```python
from build123d import *

# Parameters (mm, degrees)
F0_W          = 39
F0_H          = 51
F1_DEPTH      = 6
F2_R          = 1.4383077573
F3_DEPTH      = 4
F3_DEPTH_BACK = 4
F5_DEPTH      = 2
F6_W          = 39
F6_H          = 2.9835407734
F6_H_2        = 3.1214025915
F7_DEPTH      = 37
F8_SIZE       = 7
F9_T1_DEPTH   = 61
F10_W         = 13
F10_H         = 22
F11_DEPTH     = 15.8


# Not quite as in the source:
# - a fillet or chamfer that OpenCascade refuses, or shapes differently, is made with other operations: its cross-section is extruded or revolved along the edge and cut away or added
# - a pattern or mirror of a feature is missing from the dataset's text; its kind, count and spacing are read off the source's solid


with BuildPart() as f1:
    # F0 (on Top) → F1 (new body)
    with BuildSketch(Plane.XY):
        Rectangle(F0_W, F0_H)
    extrude(amount=F1_DEPTH)

    # F2 (on Front) → F3 (join, two sides)
    with BuildSketch(Plane.XZ) as f3_sk:
        with BuildLine():
            Line((-2.7218379916, 29.2536051472), (-13.5, 6))
            Line((-13.5, 6), (13.5, 6))
            Line((13.5, 6), (2.7218379916, 29.2536051472))
            ThreePointArc((2.7218379916, 29.2536051472), (0, 30.9920196576), (-2.7218379916, 29.2536051472))
        make_face()
        with Locations((0, 27.9920196576)):
            Circle(F2_R, mode=Mode.SUBTRACT)
    extrude(amount=F3_DEPTH)
    extrude(f3_sk.sketch, amount=-F3_DEPTH_BACK)

    # F4 (on face) → F5 (cut)
    with BuildSketch(Plane.XZ.offset(4)):
        with BuildLine():
            Line((-2.3500163027, 26.2716104284), (-11.7460088804, 6))
            Line((-11.7460088804, 6), (11.7170447484, 6))
            Line((11.7170447484, 6), (2.3322070272, 26.2475441144))
            ThreePointArc((2.3322070272, 26.2475441144), (-0.0149696172, 25.0796047749), (-2.3500163027, 26.2716104284))
        make_face()
    f5 = extrude(amount=-F5_DEPTH, mode=Mode.SUBTRACT)

    # F5_copies: F5 across plane
    add(f5.mirror(Plane.ZX), mode=Mode.SUBTRACT)

    # F6 (on face) → F7 (join)
    with BuildSketch(Plane.XY.offset(6)):
        with Locations((0, 24.0082296133)):
            Rectangle(F6_W, F6_H)
        with Locations((0, -23.9392987043)):
            Rectangle(F6_W, F6_H_2)
    extrude(amount=F7_DEPTH)

    # F8
    f8_edges = [f1.edges().sort_by_distance(p)[0] for p in [
        (19.5, 24.00823, 43),
        (-19.5, 24.00823, 43),
        (-19.5, -23.939299, 43),
        (19.5, -23.939299, 43),
    ]]
    chamfer(f8_edges, length=F8_SIZE)

    # F9: fillet of radius 5 on 4 edges, made by hand

    # F9_s2 → F9_t1 (cut)
    with BuildSketch(Plane.XY.offset(-12.5)):
        with BuildLine():
            ThreePointArc((19.5, -20.5), (18.0355339059, -24.0355339059), (14.5, -25.5))
            Line((14.5, -25.5), (19.5, -25.5))
            Line((19.5, -25.5), (19.5, -20.5))
        make_face()
        with BuildLine():
            ThreePointArc((-19.5, -20.5), (-18.0355339059, -24.0355339059), (-14.5, -25.5))
            Line((-14.5, -25.5), (-19.5, -25.5))
            Line((-19.5, -25.5), (-19.5, -20.5))
        make_face()
        with BuildLine():
            ThreePointArc((14.5, 25.5), (18.0355339059, 24.0355339059), (19.5, 20.5))
            Line((19.5, 20.5), (19.5, 25.5))
            Line((19.5, 25.5), (14.5, 25.5))
        make_face()
        with BuildLine():
            ThreePointArc((-14.5, 25.5), (-18.0355339059, 24.0355339059), (-19.5, 20.5))
            Line((-19.5, 20.5), (-19.5, 25.5))
            Line((-19.5, 25.5), (-14.5, 25.5))
        make_face()
    extrude(amount=F9_T1_DEPTH, mode=Mode.SUBTRACT)

    # F10 (on face) → F11 (cut)
    with BuildSketch(Plane(origin=(0, 25.5, 0), x_dir=(-1, 0, 0), z_dir=(0, 1, 0))):
        with Locations((0.5753570557, 27)):
            Rectangle(F10_W, F10_H)
    extrude(amount=-F11_DEPTH, mode=Mode.SUBTRACT)


solid = f1.part
```
For this review, take the finished solid that the model builds, in its own axes (mm). A direction names the side the tool comes from. Coordinates: 2 decimals unless noted, no trailing zeros. Write each loop counter-clockwise with the first axis right and the second up, starting at its lowest first coordinate (ties: lowest second). Pieces come first, ordered by that corner, then holes.
(1) Add section C-C on x = -5. Give the boundary of the cut face in (y, z).
(2) Tool access review of faces 4 (the face through (-17.413, -24.564, 20.213)), 5 (the face through (-6.98, 3.01, 16.28)), 6 (the face through (-9, 22.516, 24)), 7 (the face through (5.925, 24, 27)): name each direction out of +Z, -Z, +X, -X, +Y, -Y from which nothing blocks a thin tool from reaching the whole face with its end or side.
(3) Add section D-D on y = -18. Give the boundary of the cut face in (x, z).
(4) Add section A-A on x = 0. Give the boundary of the cut face in (y, z), then the cut area to 3 significant figures.
(5) Add section B-B on z = 13.5. Give the boundary of the cut face in (x, y), then the cut area to 3 significant figures.
(6) Wall thickness on probe 1 along Y at (x, z) = (-1.5, 6.5); probe 2 along Y at (x, z) = (9.5, 14); probe 3 along Z at (x, y) = (0, -1): over which ranges is each line inside the solid? List them lowest first.
(7) For pin 1 Ø7.5 at (x, z) = (-1, 22.5) entering from +Y; pin 2 Ø10 at (y, z) = (-7.5, 33) entering from -X; pin 3 Ø0.9 at (y, z) = (23.5, 32) entering from +X, all flat-tipped, find the tip position at first contact; note any pin that passes through.
(8) The part is to be moulded in two halves that separate along Z. For faces 1 (the face through (19.5, 0, 3)), 2 (the face through (0, 24, 43)), 3 (the face through (-7.075, 24, 27)), say which applies: +Z half, -Z half, draft (parallel to the pull), parting line (faces both ways), or undercut.
Answer sheet:
1. outline: (-25.5, 0) - (25.5, 0) - (25.5, 16) - (22.52, 16) - (22.52, 6) - (2, 6) - (2, 20.55) - (4, 20.55) - (4, 24.34) - (-4, 24.34) - (-4, 20.55) - (-2, 20.55) - (-2, 6) - (-22.38, 6) - (-22.38, 43) - (-25.5, 43) - close; (22.52, 38) - (25.5, 38) - (25.5, 43) - (22.52, 43) - close
2. face 4: +Z, -Z, -X, -Y
2. face 5: none
2. face 6: +Z, +X, -X
2. face 7: +Y
3. outline: (-19.5, 0) - (19.5, 0) - (19.5, 6) - (-19.5, 6) - close
4. outline: (-25.5, 0) - (25.5, 0) - (25.5, 16) - (22.52, 16) - (22.52, 6) - (2, 6) - (2, 25.08) - (4, 25.08) - (4, 26.55) - (-4, 26.55) - (-4, 25.08) - (-2, 25.08) - (-2, 6) - (-22.38, 6) - (-22.38, 43) - (-25.5, 43) - close; (-4, 29.43) - (4, 29.43) - (4, 30.99) - (-4, 30.99) - close; (22.52, 38) - (25.5, 38) - (25.5, 43) - (22.52, 43) - close
4. area: 567 mm2
5. outline: (-19.13, -22.38) arc R5 ccw to (-14.5, -25.5) - (14.5, -25.5) arc R5 ccw to (19.13, -22.38) - close; (-19.08, 22.52) - (19.08, 22.52) arc R5 ccw to (14.5, 25.5) - (-14.5, 25.5) arc R5 ccw to start; (-10.02, -4) - (-8.27, -4) - (-8.27, -2) - (8.24, -2) - (8.24, -4) - (10.02, -4) - (10.02, 4) - (8.24, 4) - (8.24, 2) - (-8.27, 2) - (-8.27, 4) - (-10.02, 4) - close
5. area: 312 mm2
6. probe 1: y = -25.5 to -22.38, -2 to 2, 22.52 to 25.5
6. probe 2: y = -25.5 to -22.38, -4 to 4, 22.52 to 25.5
6. probe 3: z = 0 to 26.55, 29.43 to 30.99
7. pin 1: stops at y = 4
7. pin 2: stops at x = -2.63
7. pin 3: stops at x = 18.8
8. face 1: draft
8. face 2: +Z half
8. face 3: undercut
